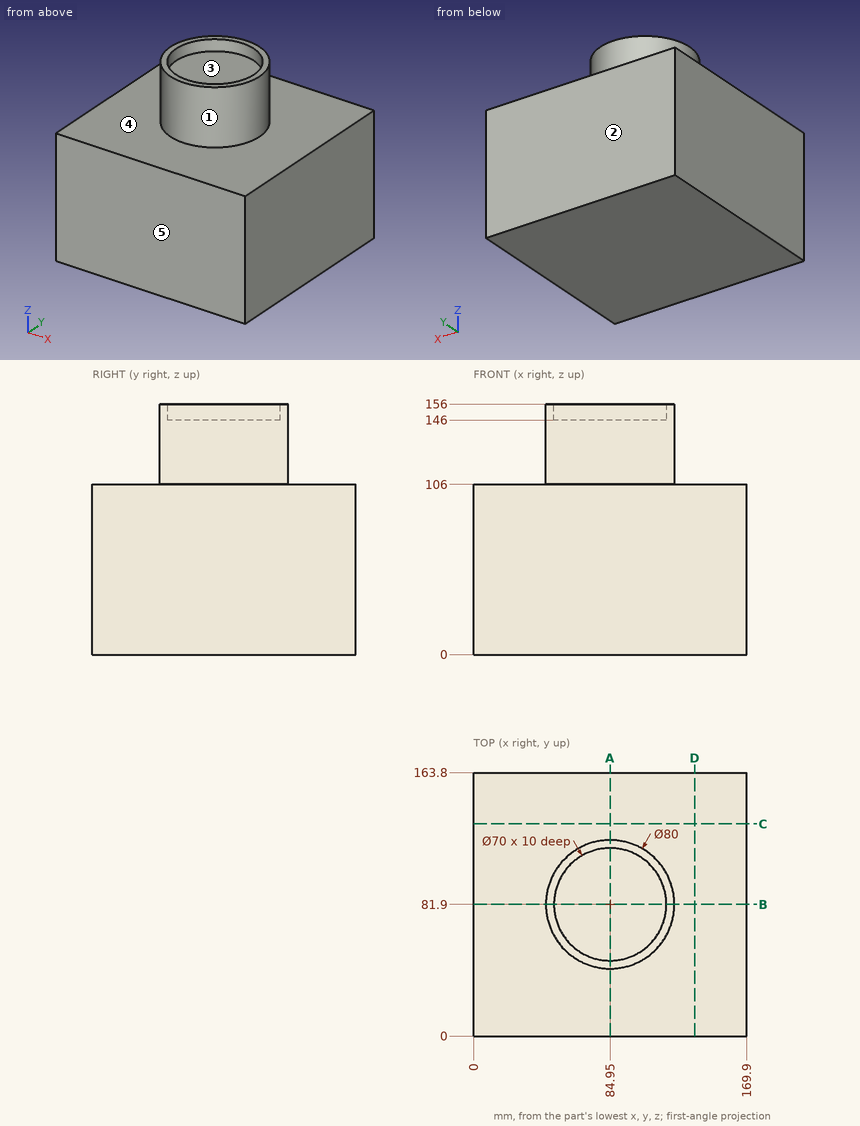
Here's the drawing with two shaded views (mm, measured from the low corner). I have some questions. A direction names the side the tool comes from. Round coordinates to 2 decimals unless told otherwise and drop trailing zeros. Loops run counter-clockwise (first coordinate to the right, second up) from the corner with the lowest first, then second, coordinate; pieces in that order, holes last. Notation, with made-up numbers: (68, -21) - (72, -21) arc R15 cw to (72, 8) - close; hole circle Ø5 at (-21.5, 50.25). An arc over 180 degrees is marked (long way). Write item = value, one per line.
1) Imagine slicing it at B-B (y = 81.9). Please give me the cut outline in (x, z), and give its area (3 significant figures).
Computed:
outline = (0, 0) - (169.9, 0) - (169.9, 106) - (124.95, 106) - (124.95, 156) - (119.95, 156) - (119.95, 146) - (49.95, 146) - (49.95, 156) - (44.95, 156) - (44.95, 106) - (0, 106) - close
area = 21,300 mm2
2) If we mould it in two halves opening along Y, with no side actions, what happens to the marked faces 1, 2 and 3? For each: pulls with the +Y half, pulls with the -Y half, needs draft (parallel to the pull), parting line crosses it, or undercut.
Computed:
face_1 = parting line crosses it
face_2 = pulls with the +Y half
face_3 = undercut
3) I need wall thicknesses on line 1 along Y through (x, z) = (84, 153); line 2 along Z through (x, y) = (66, 151.5); line 3 along X through (y, z) = (58, 107.5). Which ranges of each line are inside material? Lowest first, please. Write a range as from..to.
Computed:
line_1 = 41.91..46.91, 116.89..121.89
line_2 = 0..106
line_3 = 52.88..117.02
4) Imagine slicing it at D-D (x = 137.5). Please give me the cut outline in (y, z).
Computed:
outline = (0, 0) - (163.8, 0) - (163.8, 106) - (0, 106) - close
5) Imagine slicing it at A-A (x = 84.95). Please give me the cut outline in (y, z).
Computed:
outline = (0, 0) - (163.8, 0) - (163.8, 106) - (121.9, 106) - (121.9, 156) - (116.9, 156) - (116.9, 146) - (46.9, 146) - (46.9, 156) - (41.9, 156) - (41.9, 106) - (0, 106) - close
6) Imagine slicing it at C-C (y = 132). Please give me the cut outline in (x, z), and give its area (3 significant figures).
Computed:
outline = (0, 0) - (169.9, 0) - (169.9, 106) - (0, 106) - close
area = 18,000 mm2
7) On a 3-axis mill with a long thin cutter (end or side, diameter ignored), from which of +Z, -Z, +X, -X, +Y, -Y can I reach the whole of each face in a straight line? I mean the marked faces 4 and 5. Say none if no direction works.
Computed:
face_4 = +Z
face_5 = +Z, -Z, +X, -X, -Y
